Autodesk Inventor part; units mm, degrees
ref_plane "YZ Plane" through (0, 0, 0) normal (1, 0, 0) x (0, 1, 0)
ref_plane "XZ Plane" through (0, 0, 0) normal (0, 1, 0) x (-1, 0, 0)
ref_plane "XY Plane" through (0, 0, 0) normal (0, 0, 1) x (1, 0, 0)
sketch "Sketch1" plane through (0, 0, 0) normal (0, 1, 0) x (-1, 0, 0)
  circle A0 centre (0, 0) radius 1.5
  dimension "d0" = 3
extrude "Extrusion1" add sketch "Sketch1" along normal blind 5
sketch "Sketch2" plane through (0, 5, 0) normal (0, 1, 0) x (1, 0, 0)
  circle A0 centre (0, 0) radius 4
  dimension "d3" = 8
extrude "Extrusion2" add sketch "Sketch2" along normal blind 30
sketch "Sketch3" plane through (0, 35, 0) normal (0, 1, 0) x (1, 0, 0)
  circle A0 centre (0, 0) radius 1.5
  circle A1 centre (0, 0) radius 1.6
  dimension "d6" = 3.2
extrude "Extrusion3" cut sketch "Sketch3" against normal blind 2.5 contours A0 | A1
properties part number "ControlPanel_longStands"
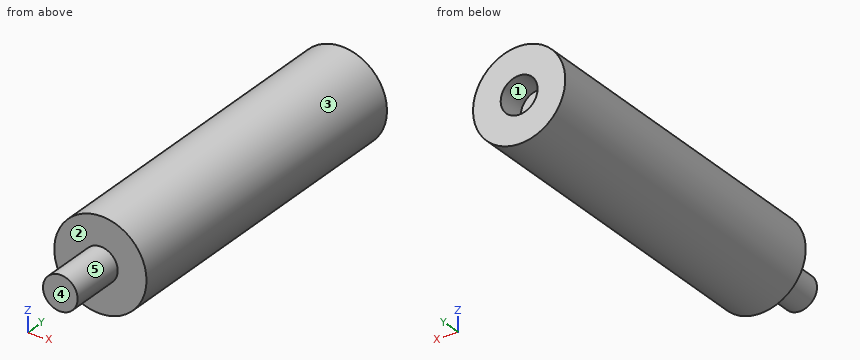
Can you work these out from the model? Positions are in its coordinate system, mm. Face numbers are marked on the shaded views. A direction names the side the tool comes from. Round coordinates to 2 decimals unless told otherwise and drop trailing zeros. Write each loop counter-clockwise with the first axis right and the second up, starting at its lowest first coordinate (ties: lowest second). Pieces come first, ordered by that corner, then holes. Notation, with made-up numbers: (75, 34) -> (132, 34) arc R21 ccw to (132, 38) -> close; hole circle Ø8 at (-34.5, 29.5). An arc over 180 degrees is marked (long way). One line per question, with ' | ' between items. Start each with the question number.
1) Suppose I cut it at C-C on y = 28.5. Write out the boundary of the cut face in (x, z).
2) On a 3-axis mill with a long thin cutter (end or side, diameter ignored), from which of +Z, -Z, +X, -X, +Y, -Y can I reach the whole of each face in a straight line? I mean the marked faces 4 and 5. Say none if no direction works.
3) If we mould it in two halves opening along Z, with no side actions, what happens to the marked faces 1, 2 and 3? For each: released by +Z, released by -Z, zero draft, split by the parting line, or undercut.
4) I need wall thicknesses on line 1 (X direction, y = 34.35, z = 0); line 2 (Y direction, x = 2.5, z = 3). Which ranges of each line are inside material? Lowest first, please. Write a range as [from, to].
5) Suppose I cut it at D-D on x = -3.25. Write out the boundary of the cut face in (y, z).
6) Suppose I cut it at A-A on z = 0. Write out the boundary of the cut face in (x, y).
7) Suppose I cut it at B-B on x = 0. Write out the boundary of the cut face in (y, z).
8) I'm going to push flat-ended pins straight in: P1, Ø1, axis at x = -1.5, y = 16.5, coming from the +Z side; P2, Ø1.5, axis at x = 2, y = 7.5, coming from the -Z side; P3, Ø2, axis at x = -2, y = 5.5, coming from the -Z side; P4, Ø3.5, axis at x = 0, z = 0, coming from the -Y side. Where does each tip first touch, or does it pass through?
Return value:
1) outline: circle Ø8 at (0, 0)
2) face 4: +Z, -Z, +X, -X, -Y | face 5: -Y
3) face 1: undercut | face 2: zero draft | face 3: split by the parting line
4) line 1: x = [-4, -1.6], [1.6, 4] | line 2: y = [5, 35]
5) outline: (5, -2.33) -> (35, -2.33) -> (35, 2.33) -> (5, 2.33) -> close
6) outline: (-4, 5) -> (-1.5, 5) -> (-1.5, 0) -> (1.5, 0) -> (1.5, 5) -> (4, 5) -> (4, 35) -> (1.6, 35) -> (1.6, 32.5) -> (-1.6, 32.5) -> (-1.6, 35) -> (-4, 35) -> close
7) outline: (0, -1.5) -> (5, -1.5) -> (5, -4) -> (35, -4) -> (35, -1.6) -> (32.5, -1.6) -> (32.5, 1.6) -> (35, 1.6) -> (35, 4) -> (5, 4) -> (5, 1.5) -> (0, 1.5) -> close
8) P1: stops at z = 3.87 | P2: stops at z = -3.8 | P3: stops at z = -3.87 | P4: stops at y = 0
